Can you work these out from the model? Positions are in its coordinate system, mm. Coordinates: 2 decimals unless noted, no trailing zeros. Loops run counter-clockwise (first coordinate to the right, second up) from the corner with the lowest first, then second, coordinate; pieces in that order, holes last. Notation, with made-up numbers: (56.25, 31.5) -> (70.25, 31.5) arc R26 cw to (70.25, 55.5) -> close; hole circle Ø5 at (10.25, -38.75). An arc over 180 degrees is marked (long way). Use one line per item in the form item = value. Start each with the question number.
(1) Imagine slicing it at B-B (x = 3.25). List the corners of the cut face in (y, z) for me, plus the area to 3 significant figures.
(2) Imagine slicing it at A-A (y = 0.4). List the corners of the cut face in (x, z) for me, plus the area to 3 significant figures.
(3) Imagine slicing it at C-C (z = -5). List the corners of the cut face in (x, y) for me, plus the area to 3 significant figures.
(4) I need wall thicknesses on line 1 (X direction, y = 0.25, z = 0); line 2 (X direction, y = 0.2, z = -7.5); line 3 (Z direction, x = -0.25, y = 0.45). Which ranges of each line are inside material? Lowest first, please. Write a range as [from, to].
(5) Thinking about a two-plate mould opening in Z: for faces 1 (the cylindrical face through (-1, 0.25, -1.31)), 2 (the flat face through (2, 0, -2)), 3 (the cylindrical face through (-2.859, 0.246, 2.797)), which applies, released by +Z, released by -Z, zero draft, split by the parting line, or undercut?
```python
from build123d import *

# Parameters (mm, degrees)
SKETCH1_R           = 1.65
BOSS_EXTRUDE1_DEPTH = 0.5


with BuildPart() as part:
    # Sketch1 → Boss-Extrude1 (new body)
    with BuildSketch(Plane(origin=(0, 0, 0), x_dir=(1, 0, 0), z_dir=(0, 1, 0))):
        with BuildLine():
            Line((11, -3.99967418), (11, 3))
            Line((11, 3), (3, 3))
            Line((3, 3), (3, 11))
            Line((3, 11), (-3.99967418, 11))
            Line((-3.99967418, 11), (-3.99967418, 0))
            ThreePointArc((-3.99967418, 0), (-2.828196736, -2.828196736), (0, -3.99967418))
            Line((0, -3.99967418), (11, -3.99967418))
        make_face()
        with Locations(Location((0, 0, 0), (0, 0, 270))):
            Circle(SKETCH1_R, mode=Mode.SUBTRACT)
    extrude(amount=BOSS_EXTRUDE1_DEPTH)


solid = part.part
```
Worked out:
q1.outline = (0, -3) -> (0.5, -3) -> (0.5, 4) -> (0, 4) -> close
q1.area = 3.50 mm2
q2.outline = (-4, -11) -> (3, -11) -> (3, -3) -> (11, -3) -> (11, 4) -> (0, 4) arc R4 ccw to (-4, 0) -> close; hole circle Ø3.3 at (0, 0)
q2.area = 149 mm2
q3.outline = (-4, 0) -> (3, 0) -> (3, 0.5) -> (-4, 0.5) -> close
q3.area = 3.50 mm2
q4.line_1 = [-4, -1.65], [1.65, 11]
q4.line_2 = [-4, 3]
q4.line_3 = [-11, -1.63], [1.63, 3.99]
q5.face_1 = undercut
q5.face_2 = zero draft
q5.face_3 = released by +Z
